Build history of the part. All positions in model axes, mm. A direction names the side the tool comes from. Give positions to 0.01 mm unless a question says otherwise; leave off trailing zeros. Loops run counter-clockwise (first coordinate to the right, second up) from the corner with the lowest first, then second, coordinate; pieces in that order, holes last. Notation, with made-up numbers: M -21,62 L 21,62 A16 cw 21,84 Z; hole C -11,-19 d5. An arc over 180 degrees is marked long. Put each result on its own line as item: value.
Autodesk Inventor part; units mm, degrees
ref_plane "Work Plane1" through (24, 0, 0) normal (1, 0, 0) x (0, 0, -1)
ref_plane "YZ Plane" through (0, 0, 0) normal (1, 0, 0) x (0, 1, 0)
ref_plane "XZ Plane" through (0, 0, 0) normal (0, 1, 0) x (-1, 0, 0)
sketch "Sketch1" plane through (0, 0, 0) normal (1, 0, 0) x (0, 1, 0)
  line L0 (21.25, 21.25) -> (-21.25, 21.25)
  line L1 (-21.25, 21.25) -> (-21.25, -21.25)
  line L2 (-21.25, -21.25) -> (21.25, -21.25)
  line L3 (21.25, -21.25) -> (21.25, 21.25)
  line L4 (21.25, 21.25) -> (-21.25, -21.25) construction
  line L5 (-21.25, 21.25) -> (21.25, -21.25) construction
  point P0 (0, 0)
  dimension "d0" = 42.5
  dimension "d1" = 42.5
extrude "Extrusion1" add sketch "Sketch1" along normal blind 8.75
chamfer "Chamfer1" distance 5 angle 45 4 edges at (4.375, 21.25, 21.25) (4.375, 21.25, -21.25) (4.375, -21.25, 21.25) (4.375, -21.25, -21.25)
sketch "Sketch2" plane through (8.75, 0, 0) normal (1, 0, 0) x (0, 0, -1)
  line L0 (21.15, -21.15) -> (-21.15, -21.15)
  line L1 (-21.15, -21.15) -> (-21.15, 21.15)
  line L2 (-21.15, 21.15) -> (21.15, 21.15)
  line L3 (21.15, 21.15) -> (21.15, -21.15)
  line L4 (21.15, -21.15) -> (-21.15, 21.15) construction
  line L5 (-21.15, -21.15) -> (21.15, 21.15) construction
  point P0 (0, 0)
  dimension "d7" = 42.3
  dimension "d8" = 42.3
extrude "Extrusion2" add sketch "Sketch2" along normal blind 30.5
chamfer "Chamfer2" distance 8 angle 45 4 edges at (24, 21.15, 21.15) (24, 21.15, -21.15) (24, -21.15, 21.15) (24, -21.15, -21.15)
ref_plane "Work Plane1" through (24, 0, 0) normal (1, 0, 0) x (0, 0, -1)
mirror "Mirror1" about plane through (24, 0, 0) normal (1, 0, 0) of "Extrusion1"
chamfer "Chamfer3" distance 5 angle 45 4 edges at (43.625, 21.25, -21.25) (43.625, -21.25, -21.25) (43.625, -21.25, 21.25) (43.625, 21.25, 21.25)
sketch "Sketch3" plane through (48, -16.25, 21.25) normal (1, 0, 0) x (0, 0, -1)
  point P0 (21.25, 16.25)
  point P1 (36.75, 31.75)
  point P2 (36.75, 0.75)
  point P3 (5.75, 0.75)
  point P4 (5.75, 31.75)
  dimension "d17" = 31
  dimension "d18" = 31
  dimension "d19" = 15.5
  dimension "d20" = 15.5
hole "Hole1" at (48, 15.5, -15.5) at (48, -15.5, -15.5) at (48, -15.5, 15.5) at (48, 15.5, 15.5) direction (-1, 0, 0) diameter 2.459 depth 18 tip angle 118
sketch "Sketch4" plane through (48, -16.25, 21.25) normal (1, 0, 0) x (0, 0, -1)
  circle A0 centre (21.25, 16.25) radius 11
  dimension "d28" = 22
extrude "Extrusion3" add sketch "Sketch4" along normal blind 2
sketch "Sketch5" plane through (50, 0, 0) normal (1, 0, 0) x (0, 0, -1)
  circle A0 centre (0, 0) radius 2.5
  dimension "d31" = 5
extrude "Extrusion4" add sketch "Sketch5" along normal blind 22
sketch "Sketch6" plane through (72, 0, 0) normal (1, 0, 0) x (0, 0, -1)
  circle A0 centre (0, 0) radius 2.5
  line L0 (2, 1.5) -> (2, -1.5)
  point P0 (2, 0)
  dimension "d34" = 2
extrude "Extrusion5" cut sketch "Sketch6" against normal blind 20 contours A0 L0 picked at (2.0912, -0.3466)
equation "\"d1\" = d0"
equation "\"d8\" = d7"
properties part number "HCMUTE-CDT23-OP_STEP-42"
Q1. Mould opens along Y. For faces 1 (the flat face through (4, 0, 21.25)), 2 (the flat face through (4.3, 18.7, -18.8)), 3 (the cylindrical face through (38.874, -15.869, -16.673)) say: pulls with the +Y half, pulls with the -Y half, needs draft (parallel to the pull), parting line crosses it, or undercut.
Here are the results:
face 1: needs draft
face 2: pulls with the +Y half
face 3: undercut
Q2. Slice it at D-D (x = 19.5). List the corners of the cut face in (y, z).
Here are the results:
outline: M -21.15,-13.15 L -13.15,-21.15 L 13.15,-21.15 L 21.15,-13.15 L 21.15,13.15 L 13.15,21.15 L -13.15,21.15 L -21.15,13.15 Z
Q3. Slice it at A-A (z = 0). List the corners of the cut face in (x, y).
Here are the results:
outline: M 0,-21.25 L 8.75,-21.25 L 8.75,-21.15 L 39.25,-21.15 L 39.25,-21.25 L 48,-21.25 L 48,-11 L 50,-11 L 50,-2.5 L 72,-2.5 L 72,2.5 L 50,2.5 L 50,11 L 48,11 L 48,21.25 L 39.25,21.25 L 39.25,21.15 L 8.75,21.15 L 8.75,21.25 L 0,21.25 Z
Q4. Probe line 1 (Z direction, x = 43.5, y = -15.5); line 2 (Z direction, x = 34, y = 15). List the from-to ranges inside material, lowest first. Write a range as from..to.
Here are the results:
line 1: -21.25..-16.73, -14.27..14.27, 16.73..21.25
line 2: -19.3..-16.62, -14.38..14.38, 16.62..19.3
Q5. Slice it at C-C (x = 31.5). List the corners of the cut face in (y, z).
Here are the results:
outline: M -21.15,-13.15 L -13.15,-21.15 L 13.15,-21.15 L 21.15,-13.15 L 21.15,13.15 L 13.15,21.15 L -13.15,21.15 L -21.15,13.15 Z; hole C -15.5,-15.5 d2.46; hole C -15.5,15.5 d2.46; hole C 15.5,-15.5 d2.46; hole C 15.5,15.5 d2.46
Q6. Tool access for faces 4 (the cylindrical face through (60.8, -0.1, 2.5)), 5 (the flat face through (23.8, -17.2, -17.1)), 6 (the flat face through (24, 0, -21.15)), 7 (the flat face through (23.8, -17.2, 17.1)): list every direction of +Z, -Z, +X, -X, +Y, -Y with a clear straight run to the whole face (end or side of a thin tool).
Here are the results:
face 4: +X
face 5: -Z, -Y
face 6: -Z, +Y, -Y
face 7: +Z, -Y
Q7. Slice it at B-B (y = 0). List the corners of the cut face in (x, z).
Here are the results:
outline: M 0,-21.25 L 8.75,-21.25 L 8.75,-21.15 L 39.25,-21.15 L 39.25,-21.25 L 48,-21.25 L 48,-11 L 50,-11 L 50,-2.5 L 52,-2.5 L 52,-2 L 72,-2 L 72,2.5 L 50,2.5 L 50,11 L 48,11 L 48,21.25 L 39.25,21.25 L 39.25,21.15 L 8.75,21.15 L 8.75,21.25 L 0,21.25 Z
Q8. Drop flat-ended pins along their axis: pin 1 Ø12 at (x, z) = (28.5, -10) entering from +Y; pin 2 Ø2 at (y, z) = (15.5, -15.5) entering from +X; pin 3 Ø1.5 at (x, y) = (62.5, 0.5) entering from -Z. Give the stop position or say it passes through.
Here are the results:
pin 1: y = 21.15
pin 2: x = 29.86
pin 3: z = -2
